The model under review builds one solid part; all positions refer to its coordinate system, in mm. Round coordinates to 2 decimals unless told otherwise and drop trailing zeros. Order: outer loops, then holes, each group sorted by start corner. A loop starts at its lowest first (then second) coordinate and runs counter-clockwise, first axis right, second up. Notation, with made-up numbers: M 49.25,4 L 63.25,4 A24 cw 63.25,30 Z; hole C 23,75 d8. An arc over 180 degrees is marked long. One line per item, written item: value. Start each with the question number.
Autodesk Inventor part; units mm, degrees
ref_plane "YZ Plane" through (0, 0, 0) normal (1, 0, 0) x (0, 1, 0)
ref_plane "XZ Plane" through (0, 0, 0) normal (0, 1, 0) x (-1, 0, 0)
ref_plane "XY Plane" through (0, 0, 0) normal (0, 0, 1) x (1, 0, 0)
sketch "Sketch9" plane through (0, 0, 0) normal (0, 1, 0) x (-1, 0, 0)
  line L0 (0, 0) -> (-250, 0)
  line L1 (-250, 0) -> (-250, -86.6623)
  line L2 (-250, -86.6623) -> (0, -86.6623)
  line L3 (0, -86.6623) -> (0, 0)
  dimension "d59" = 86.6623
  dimension "d60" = 250
extrude "Extrusion5" add sketch "Sketch9" along normal blind 3.2
sketch "Sketch10" plane through (0, 3.2, 0) normal (0, 1, 0) x (1, 0, 0)
  line L0 (22, 0) -> (103.05, 0)
  line L1 (103.05, 0) -> (103.05, 34.3311)
  line L2 (103.05, 34.3311) -> (22, 34.3311)
  line L3 (22, 34.3311) -> (22, 0)
  line L4 (250, 86.6623) -> (0, 86.6623)
  line L5 (103.05, 86.6623) -> (22, 86.6623)
  line L6 (22, 86.6623) -> (22, 52.3311)
  line L7 (22, 52.3311) -> (103.05, 52.3311)
  line L8 (103.05, 52.3311) -> (103.05, 86.6623)
  line L9 (0, 0) -> (250, 0)
  line L10 (0, 86.6623) -> (0, 0)
  dimension "d63" = 22
  dimension "d64" = 34.3311
  dimension "d65" = 81.05
  dimension "d66" = 34.3311
extrude "Extrusion6" cut sketch "Sketch10" against normal blind 3.2
sketch "Sketch11" plane through (0, 3.2, 0) normal (0, 1, 0) x (1, 0, 0)
  line L0 (237.05, 7.3311) -> (136.05, 7.3311)
  line L1 (136.05, 7.3311) -> (136.05, 79.3311)
  line L2 (136.05, 79.3311) -> (237.05, 79.3311)
  line L3 (237.05, 79.3311) -> (237.05, 7.3311)
  line L4 (103.05, 86.6623) -> (103.05, 52.3311)
  line L5 (0, 86.6623) -> (0, 0)
  line L6 (103.05, 0) -> (250, 0)
  line L7 (121.05, 0) -> (121.05, 86.188) construction
  line L8 (103.05, 34.3311) -> (103.05, 0)
  line L9 (240.25, 4.1311) -> (132.85, 4.1311)
  line L10 (132.85, 4.1311) -> (132.85, 82.5311)
  line L11 (132.85, 82.5311) -> (240.25, 82.5311)
  line L12 (240.25, 82.5311) -> (240.25, 4.1311)
  dimension "d69" = 72
  dimension "d70" = 101
  dimension "d71" = 33
  dimension "d72" = 86.6623
  dimension "d73" = 7.3311
  dimension "d74" = 18
  dimension "d75" = 3.2
  dimension "d76" = 3.2
  dimension "d77" = 3.2
  dimension "d78" = 3.2
extrude "Extrusion7" cut sketch "Sketch11" against normal blind 1
sketch "Sketch12" plane through (0, 3.2, 0) normal (0, 1, 0) x (1, 0, 0)
  line L0 (237.05, 7.3311) -> (237.05, 79.3311)
  line L1 (237.05, 79.3311) -> (136.05, 79.3311)
  line L2 (136.05, 79.3311) -> (136.05, 7.3311) construction
  line L3 (136.05, 7.3311) -> (237.05, 7.3311)
  line L4 (144.05, 15.3311) -> (229.05, 15.3311) construction
  line L5 (229.05, 15.3311) -> (229.05, 71.3311) construction
  line L6 (229.05, 71.3311) -> (144.05, 71.3311) construction
  line L7 (144.05, 71.3311) -> (144.05, 15.3311) construction
  line L8 (152.05, 15.3311) -> (144.05, 23.3311)
  line L9 (144.05, 23.3311) -> (144.05, 31.3311)
  line L10 (144.05, 31.3311) -> (160.05, 15.3311)
  line L11 (160.05, 15.3311) -> (152.05, 15.3311)
  line L12 (169.9495, 15.3311) -> (144.05, 41.2306)
  line L13 (144.05, 41.2306) -> (144.05, 49.2306)
  line L14 (144.05, 49.2306) -> (177.9495, 15.3311)
  line L15 (169.9495, 15.3311) -> (177.9495, 15.3311)
  line L16 (187.849, 15.3311) -> (144.05, 59.1301)
  line L17 (144.05, 59.1301) -> (144.05, 67.1301)
  line L18 (144.05, 67.1301) -> (195.849, 15.3311)
  line L19 (195.849, 15.3311) -> (187.849, 15.3311)
  line L20 (213.7485, 15.3311) -> (205.7485, 15.3311)
  line L21 (157.7485, 71.3311) -> (213.7485, 15.3311)
  line L22 (223.648, 15.3311) -> (167.648, 71.3311)
  line L23 (185.5475, 71.3311) -> (193.5475, 71.3311)
  line L24 (193.5475, 71.3311) -> (229.05, 35.8286)
  line L25 (229.05, 45.7281) -> (203.447, 71.3311)
  line L26 (203.447, 71.3311) -> (211.447, 71.3311)
  line L27 (229.05, 63.6276) -> (221.3465, 71.3311)
  line L28 (229.05, 45.7281) -> (229.05, 53.7281)
  line L29 (229.05, 53.7281) -> (211.447, 71.3311)
  line L30 (205.7485, 15.3311) -> (149.7485, 71.3311)
  line L31 (149.7485, 71.3311) -> (157.7485, 71.3311)
  line L32 (185.5475, 71.3311) -> (229.05, 27.8286)
  line L33 (229.05, 27.8286) -> (229.05, 35.8286)
  line L34 (223.648, 15.3311) -> (229.05, 15.3311)
  line L35 (229.05, 15.3311) -> (229.05, 17.9291)
  line L36 (229.05, 17.9291) -> (175.648, 71.3311)
  line L37 (167.648, 71.3311) -> (175.648, 71.3311)
  line L38 (229.05, 63.6276) -> (229.05, 71.3311)
  line L39 (229.05, 71.3311) -> (221.3465, 71.3311)
  point P0 (0, 0)
  dimension "d81" = 8
  dimension "d82" = 8
  dimension "d83" = 8
  dimension "d84" = 8
  dimension "d85" = 8
  dimension "d86" = 8
  dimension "d88" = 7
  dimension "d90" = 7
  dimension "d92" = 7
  dimension "d95" = 7
  dimension "d97" = 7
  dimension "d98" = 7
  dimension "d100" = 7
extrude "Extrusion8" cut sketch "Sketch12" against normal up to surface (3.2 mm away)
sketch "Sketch13" plane through (0, 3.2, 0) normal (0, 1, 0) x (1, 0, 0)
  circle A0 centre (116.05, 5) radius 2.5
  circle A1 centre (116.05, 81.6623) radius 2.5
  circle A2 centre (40.35, 43.3311) radius 2.5
  circle A3 centre (80.7, 43.3311) radius 2.5
  line L0 (0, 86.6623) -> (0, 0)
  line L1 (103.05, 0) -> (250, 0)
  line L2 (103.05, 34.3311) -> (103.05, 0)
  line L3 (250, 86.6623) -> (103.05, 86.6623)
  circle A4 centre (8, 15.25) radius 2.5
  circle A5 centre (8, 71.4123) radius 2.5
  line L4 (0, 0) -> (22, 0)
  line L5 (22, 86.6623) -> (0, 86.6623)
  point P0 (0, 43.3311)
  dimension "d103" = 40.35
  dimension "d104" = 40.35
  dimension "d105" = 5
  dimension "d106" = 5
  dimension "d107" = 13
  dimension "d108" = 5
  dimension "d109" = 15.25
  dimension "d110" = 15.25
  dimension "d111" = 8
extrude "Extrusion9" cut sketch "Sketch13" against normal up to surface (3.2 mm away)
sketch "Sketch14" plane through (0, 3.2, 0) normal (0, 1, 0) x (1, 0, 0)
  line L0 (250, 0) -> (250, 86.6623)
  line L1 (103.05, 34.3311) -> (103.05, 0)
  point P0 (0, 0)
  dimension "largo_abdomen_robot" = 146.95
sketch "Sketch15" plane through (0, 3.2, 0) normal (0, 1, 0) x (1, 0, 0)
  line L0 (250, 0) -> (250, 86.6623)
  line L1 (250, 86.6623) -> (121.05, 86.6623)
  line L2 (121.05, 86.6623) -> (121.05, 89.8623)
  line L3 (121.05, 89.8623) -> (250, 89.8623)
  line L4 (250, 89.8623) -> (250, 86.6623)
  line L5 (250, 0) -> (121.05, 0)
  line L6 (121.05, 0) -> (121.05, -3.2)
  line L7 (121.05, -3.2) -> (250, -3.2)
  line L8 (250, -3.2) -> (250, 0)
  point P0 (0, 0)
  dimension "d115" = 128.95
  dimension "d116" = 3.2
extrude "Extrusion10" add sketch "Sketch15" against normal up to surface (3.2 mm away)
sketch "Sketch16" plane through (0, 3.2, 0) normal (0, 1, 0) x (1, 0, 0)
  line L0 (0, 0) -> (22, 0)
  line L1 (18, 0) -> (8, 0)
  line L2 (8, 0) -> (8, -3.2)
  line L3 (8, -3.2) -> (18, -3.2)
  line L4 (18, -3.2) -> (18, 0)
  line L5 (18, 86.6623) -> (8, 86.6623)
  line L6 (8, 86.6623) -> (8, 89.8623)
  line L7 (8, 89.8623) -> (18, 89.8623)
  line L8 (18, 89.8623) -> (18, 86.6623)
  line L9 (22, 86.6623) -> (0, 86.6623)
  line L10 (22, 0) -> (22, 34.3311)
  dimension "d119" = 4
  dimension "d120" = 10
  dimension "d121" = 3.2
extrude "Extrusion11" add sketch "Sketch16" against normal up to surface (3.2 mm away)
equation "\"d59\" = ancho_acople_hombros"
equation "\"d63\" = acople_hombro_grosor_frontal"
equation "\"d64\" = acople_hombro_ancho_agujero"
equation "\"d65\" = acople_hombro_largo_agujero"
equation "\"d66\" = acople_hombro_ancho_agujero"
equation "\"d73\" = -0.5 * d69 + 0.5 * d72"
equation "\"d74\" = acople_hombro_grosor_trasero"
equation "\"d76\" = d75"
equation "\"d77\" = d76"
equation "\"d78\" = d75"
equation "\"d82\" = d81"
equation "\"d83\" = d81"
equation "\"d84\" = d81"
equation "\"d86\" = d85"
equation "\"d88\" = d95"
equation "\"d90\" = d95"
equation "\"d92\" = d91"
equation "\"d97\" = d92"
equation "\"d98\" = d95"
equation "\"d100\" = d95"
equation "\"d103\" = dist_agujero_central_a_frente"
equation "\"d104\" = d103"
equation "\"d105\" = diametro_tornillo"
equation "\"d106\" = dist_agujero_trasero_a_lado"
equation "\"d107\" = dist_agujero_trasero_a_frente"
equation "\"d108\" = d106"
equation "\"d109\" = dist_agujero_frontal_a_lateral"
equation "\"d110\" = d109"
equation "\"d111\" = dist_agujero_frontal_a_frente"
equation "\"d115\" = largo_abdomen_robot - acople_hombro_grosor_trasero"
equation "\"d91\" = d90"
properties part number "cuerpo-base-bateria"
Item 1: Clearance check with flat-ended pins moving along their axes: P1, Ø1.6, axis at x = 6, y = 1.5, coming from the +Z side; P2, Ø1, axis at x = 59.5, y = 2.5, coming from the +Z side. State where each tip first meets the part, or that it passes through.
Item 2: The part is to be moulded in two halves that separate along X. For faces 1 (the flat face through (151.94, 1.62, -23.44)), 2 (the flat face through (187, 3.2, -43)), say which applies: pulls with the +X half, pulls with the -X half, needs draft (parallel to the pull), parting line crosses it, or undercut.
Item 3: Consider section B-B, the plane x = 80.7. Give the boundary of the cut face in (y, z).
Item 4: Wall thickness on L1, parallel to Z at x = 116.05, y = 2.25; L2, parallel to X at y = 0.7, z = -5.5; L3, parallel to X at y = 1.65, z = -15.25: over which ranges is each line inside the solid? List them lowest first.
Item 5: Consider section C-C, the plane y = 0.5. Count the separate pieces of the cut face and the enclosed holes in it, then the cut area to 3 significant figures.
Item 6: Consider section A-A, the plane x = 116.05. Give the boundary of the cut face in (y, z), then the cut area to 3 significant figures.
Computed:
1. P1: stops at z = 0
1. P2: stops at z = -34.33
2. face 1: undercut
2. face 2: needs draft
3. outline: M 0,-52.33 L 3.2,-52.33 L 3.2,-45.83 L 0,-45.83 Z; M 0,-40.83 L 3.2,-40.83 L 3.2,-34.33 L 0,-34.33 Z
4. L1: z = -86.66 to -84.16, -79.16 to -7.5, -2.5 to 0
4. L2: x = 0 to 22, 103.05 to 113.6, 118.5 to 250
4. L3: x = 0 to 5.5, 10.5 to 22, 103.05 to 250
5. separate pieces: 1
5. enclosed holes: 14
5. area: 14,700 mm^2
6. outline: M 0,-86.66 L 3.2,-86.66 L 3.2,-84.16 L 0,-84.16 Z; M 0,-79.16 L 3.2,-79.16 L 3.2,-7.5 L 0,-7.5 Z; M 0,-2.5 L 3.2,-2.5 L 3.2,0 L 0,0 Z
6. area: 245 mm^2
